The model under review builds one solid part; all positions refer to its coordinate system, in mm. Face numbers are marked on the shaded views. Round coordinates to 2 decimals unless told otherwise and drop trailing zeros. Loops run counter-clockwise (first coordinate to the right, second up) from the corner with the lowest first, then second, coordinate; pieces in that order, holes last. Notation, with made-up numbers: (-0.75, 5.5) -> (16.25, 5.5) arc R33 cw to (16.25, 44.5) -> close; hole circle Ø10 at (23.25, 59.5). An arc over 180 degrees is marked (long way). Write each question's results on one line, items separated by ' | '. Start each with the question number.
Item 1: We need section B-B (z = 7.5). Give the boundary of the cut face in (x, y).
Item 2: Mouldability with a two-part tool opening along Z and no side actions: class the marked faces 1, 2 and 3 as pulls with the +Z half, pulls with the -Z half, needs draft (parallel to the pull), parting line crosses it, or undercut.
Item 3: We need section A-A (x = -5.75). Give the boundary of the cut face in (y, z).
Item 4: Clearance check with flat-ended pins moving along their axes: pin 1 Ø2 at (y, z) = (3.5, 13) entering from -X; pin 2 Ø2 at (x, z) = (5, 8) entering from +Y; pin 3 Ø1.5 at (y, z) = (2.5, 9) entering from -X; pin 4 Ø1 at (x, y) = (6, 2.5) entering from -Z. State where each tip first meets the part, or that it passes through.
Item 5: For L1, parallel to Z at x = -6, y = 0; L2, parallel to X at y = 4.75, z = -7; L3, parallel to Y at x = -0.25, z = 5.5, list the stretches that pass through material, from the lowest coordinate up. Write a range as from..to.
Autodesk Inventor part; units mm, degrees
ref_plane "YZ Plane" through (0, 0, 0) normal (1, 0, 0) x (0, 1, 0)
ref_plane "XZ Plane" through (0, 0, 0) normal (0, 1, 0) x (-1, 0, 0)
ref_plane "XY Plane" through (0, 0, 0) normal (0, 0, 1) x (1, 0, 0)
sketch "Skizze1" plane through (0, 0, 0) normal (0, 0, 1) x (1, 0, 0)
  circle A0 centre (0, 0) radius 5
  dimension "d0" = 10
extrude "Extrusion1" add sketch "Skizze1" along normal blind 40
sketch "Skizze2" plane through (0, 0, 40) normal (0, 0, 1) x (1, 0, 0)
  circle A0 centre (0, 0) radius 5
  circle A1 centre (0, 0) radius 7.5
  circle A2 centre (0, 0) radius 5
  line L0 (0, -5) -> (-1.3746, -7.373)
  line L1 (-1.3746, -7.373) -> (-1.8625, -4.6402)
  arc A3 (-1.8625, -4.6402) -> (0, -5) centre (0, 0) ccw
  line L2 (2.1694, -4.5048) -> (1.9606, -7.2392)
  line L3 (1.9606, -7.2392) -> (0.3352, -4.9888)
  arc A4 (0.3352, -4.9888) -> (2.1694, -4.5048) centre (0, 0) ccw
  line L4 (3.9092, -3.1174) -> (4.9074, -5.6716)
  line L5 (4.9074, -5.6716) -> (2.4666, -4.3493)
  arc A5 (2.4666, -4.3493) -> (3.9092, -3.1174) centre (0, 0) ccw
  line L6 (4.8746, -1.1126) -> (6.8822, -2.9807)
  line L7 (6.8822, -2.9807) -> (4.1094, -2.8484)
  arc A6 (4.1094, -2.8484) -> (4.8746, -1.1126) centre (0, 0) ccw
  line L8 (4.8746, 1.1126) -> (7.494, 0.3005)
  line L9 (7.494, 0.3005) -> (4.9383, -0.7833)
  arc A7 (4.9383, -0.7833) -> (4.8746, 1.1126) centre (0, 0) ccw
  line L10 (3.9092, 3.1174) -> (6.6214, 3.5223)
  line L11 (6.6214, 3.5223) -> (4.7891, 1.4369)
  arc A8 (4.7891, 1.4369) -> (3.9092, 3.1174) centre (0, 0) ccw
  line L12 (2.1694, 4.5048) -> (4.4375, 6.0464)
  line L13 (4.4375, 6.0464) -> (3.6914, 3.3725)
  arc A9 (3.6914, 3.3725) -> (2.1694, 4.5048) centre (0, 0) ccw
  line L14 (0, 5) -> (1.3746, 7.373)
  line L15 (1.3746, 7.373) -> (1.8625, 4.6402)
  arc A10 (1.8625, 4.6402) -> (0, 5) centre (0, 0) ccw
  line L16 (-2.1694, 4.5048) -> (-1.9606, 7.2392)
  line L17 (-1.9606, 7.2392) -> (-0.3352, 4.9888)
  arc A11 (-0.3352, 4.9888) -> (-2.1694, 4.5048) centre (0, 0) ccw
  line L18 (-3.9092, 3.1174) -> (-4.9074, 5.6716)
  line L19 (-4.9074, 5.6716) -> (-2.4666, 4.3493)
  arc A12 (-2.4666, 4.3493) -> (-3.9092, 3.1174) centre (0, 0) ccw
  line L20 (-4.8746, 1.1126) -> (-6.8822, 2.9807)
  line L21 (-6.8822, 2.9807) -> (-4.1094, 2.8484)
  arc A13 (-4.1094, 2.8484) -> (-4.8746, 1.1126) centre (0, 0) ccw
  line L22 (-4.8746, -1.1126) -> (-7.494, -0.3005)
  line L23 (-7.494, -0.3005) -> (-4.9383, 0.7833)
  arc A14 (-4.9383, 0.7833) -> (-4.8746, -1.1126) centre (0, 0) ccw
  line L24 (-3.9092, -3.1174) -> (-6.6214, -3.5223)
  line L25 (-6.6214, -3.5223) -> (-4.7891, -1.4369)
  arc A15 (-4.7891, -1.4369) -> (-3.9092, -3.1174) centre (0, 0) ccw
  line L26 (-2.1694, -4.5048) -> (-4.4375, -6.0464)
  line L27 (-4.4375, -6.0464) -> (-3.6914, -3.3725)
  arc A16 (-3.6914, -3.3725) -> (-2.1694, -4.5048) centre (0, 0) ccw
  dimension "d3" = 15
  dimension "d6" = 360
extrude "Extrusion2" add sketch "Skizze2" along normal blind 15 contours A0 | A0 L8 L9 | A0 L10 L11 | L6 L7 A0 | A0 L12 L13 | L4 L5 A0 | L15 A0 L14 | L3 A0 L2 | L17 A0 L16 | L1 A0 L0 | L19 A0 L18 | L27 A0 L26 | L21 A0 L20 | L25 A0 L24 | L23 A0 L22
ref_plane "Arbeitsebene1" through (0, 0, 20) normal (0, 0, -1) x (-1, 0, 0)
mirror "Spiegeln2" about plane through (0, 0, 20) normal (0, 0, -1) of "Extrusion2"
equation "\"d0\" = Durchmesser3"
equation "\"d3\" = Durchmesser1"
equation "\"d8\" = Größe4"
equation "\"Durchmesser1\" = 15"
equation "\"Größe1\" = 7"
equation "\"Durchmesser2\" = 3"
equation "\"Durchmesser3\" = 10"
equation "\"Größe3\" = 3"
equation "\"Größe4\" = 15"
properties part number "WelleRuder1"
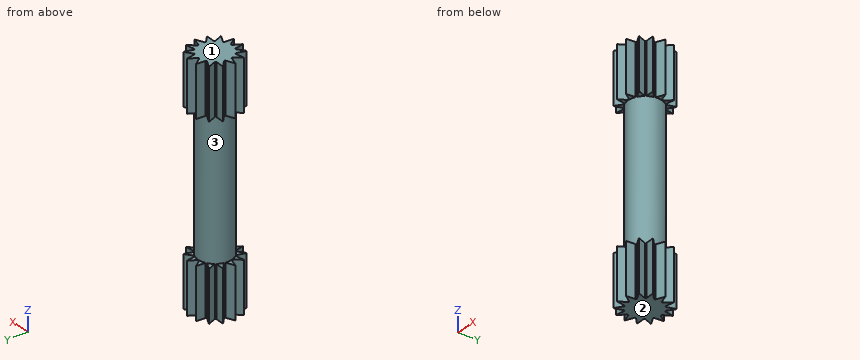
Here are the results:
1) outline: circle Ø10 at (0, 0)
2) face 1: pulls with the +Z half | face 2: pulls with the -Z half | face 3: undercut
3) outline: (-3.39, -15) -> (-2.53, -15) -> (-2.53, 0) -> (-3.39, 0) -> close; (-3.39, 40) -> (-2.53, 40) -> (-2.53, 55) -> (-3.39, 55) -> close; (-0.84, -15) -> (0.44, -15) -> (0.44, 0) -> (-0.84, 0) -> close; (-0.84, 40) -> (0.44, 40) -> (0.44, 55) -> (-0.84, 55) -> close; (1.93, -15) -> (2.93, -15) -> (2.93, 0) -> (1.93, 0) -> close; (1.93, 40) -> (2.93, 40) -> (2.93, 55) -> (1.93, 55) -> close
4) pin 1: stops at x = -4.33 | pin 2: stops at y = 3 | pin 3: stops at x = -4.68 | pin 4: stops at z = -15
5) L1: z = -15..0, 40..55 | L2: x = -4.55..-3.21, -2.15..1.84, 2.53..4.08 | L3: y = -4.99..4.99
